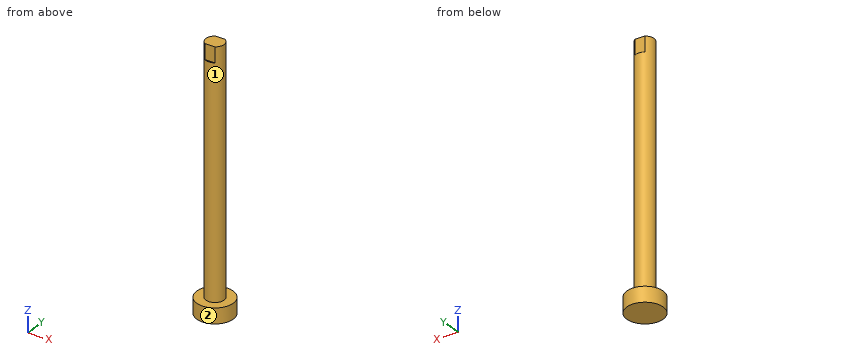
from build123d import *

# Parameters (mm, degrees)
F0_R     = 3
F1_DEPTH = 40
F2_R     = 6
F2_R_2   = 3
F3_DEPTH = 5
F5_DEPTH = 5


with BuildPart() as f1:
    # F0 (on Top) → F1 (new body, symmetric)
    with BuildSketch(Plane.XY):
        Circle(F0_R)
    extrude(amount=F1_DEPTH, both=True)

    # F2 (on face) → F3 (join)
    with BuildSketch(Plane(origin=(0, 0, -40), x_dir=(1, 0, 0), z_dir=(0, 0, -1))):
        Circle(F2_R)
        Circle(F2_R_2, mode=Mode.SUBTRACT)
        Circle(F2_R_2)
    extrude(amount=F3_DEPTH)

    # F4 (on face) → F5 (cut)
    with BuildSketch(Plane.XY.offset(40)):
        with BuildLine():
            Line((4.5341607578, -3.7982849256), (4.5341607578, -2.5))
            Line((4.5341607578, -2.5), (1.6583123952, -2.5))
            ThreePointArc((1.6583123952, -2.5), (0, -3), (-1.6583123952, -2.5))
            Line((-1.6583123952, -2.5), (-4.5341607578, -2.5))
            Line((-4.5341607578, -2.5), (-4.5341607578, -3.7982849256))
            Line((-4.5341607578, -3.7982849256), (4.5341607578, -3.7982849256))
        make_face()
        with BuildLine():
            ThreePointArc((-1.6583123952, -2.5), (0, -3), (1.6583123952, -2.5))
            Line((1.6583123952, -2.5), (-1.6583123952, -2.5))
        make_face()
        with BuildLine():
            Line((1.6583123952, 2.5), (4.5341607578, 2.5))
            Line((4.5341607578, 2.5), (4.5341607578, 3.7982849256))
            Line((4.5341607578, 3.7982849256), (-4.5341607578, 3.7982849256))
            Line((-4.5341607578, 3.7982849256), (-4.5341607578, 2.5))
            Line((-4.5341607578, 2.5), (-1.6583123952, 2.5))
            ThreePointArc((-1.6583123952, 2.5), (0, 3), (1.6583123952, 2.5))
        make_face()
        with BuildLine():
            Line((-1.6583123952, 2.5), (1.6583123952, 2.5))
            ThreePointArc((1.6583123952, 2.5), (0, 3), (-1.6583123952, 2.5))
        make_face()
    extrude(amount=-F5_DEPTH, mode=Mode.SUBTRACT)


solid = f1.part
The model under review builds one solid part; all positions refer to its coordinate system, in mm. Face numbers are marked on the shaded views. A direction names the side the tool comes from. Give positions to 0.01 mm unless a question says otherwise; leave off trailing zeros. Order: outer loops, then holes, each group sorted by start corner. A loop starts at its lowest first (then second) coordinate and runs counter-clockwise, first axis right, second up. Notation, with made-up numbers: M 68,37.5 L 109,37.5 A7 ccw 109,48.5 Z; hole C 85,49 d4. An arc over 180 degrees is marked long. Answer in a Markdown table with one row per item. Add a question column.
1. Add section C-C on z = -16. State the section outline as (x, y) points.
2. To check wall thickness, follow line 1 along Z through (x, y) = (-1.5, -4); line 2 along X through (y, z) = (2.5, 24); line 3 along X through (y, z) = (-0.25, -22). State the ranges of each line that lie inside material, in increasing order.
3. Add section B-B on x = 0. State the section outline as (y, z) points, plus the area to 3 significant figures.
4. For pin 1 Ø3.5 at (x, z) = (0.5, 38) entering from -Y; pin 2 Ø2.5 at (x, z) = (0, 38) entering from +Y; pin 3 Ø5 at (y, z) = (-0.5, 27.5) entering from +X, all flat-tipped, find the tip position at first contact; note any pin that passes through.
5. Machinability: for the marked faces 1 and 2, which of the approach directions +Z, -Z, +X, -X, +Y, -Y give a long, thin tool a straight path to every point of the face, cutting with its end or side? Answer none if there is none.
6. Add section A-A on y = 0. State the section outline as (x, z) points, plus the area to 3 significant figures.
7. Add section D-D on y = 4.75. State the section outline as (x, z) points, plus the area to 3 significant figures.
The answers:
| question | item | result |
|---|---|---|
| 1 | outline | C 0,0 d6 |
| 2 | line 1 | -45 to -40 |
| 2 | line 2 | -1.66 to 1.66 |
| 2 | line 3 | -2.99 to 2.99 |
| 3 | outline | M -6,-45 L 6,-45 L 6,-40 L 3,-40 L 3,35 L 2.5,35 L 2.5,40 L -2.5,40 L -2.5,35 L -3,35 L -3,-40 L -6,-40 Z |
| 3 | area | 535 mm2 |
| 4 | pin 1 | y = -2.5 |
| 4 | pin 2 | y = 2.5 |
| 4 | pin 3 | x = 3 |
| 5 | face 1 | +Z |
| 5 | face 2 | +Z, -Z |
| 6 | outline | M -6,-45 L 6,-45 L 6,-40 L 3,-40 L 3,40 L -3,40 L -3,-40 L -6,-40 Z |
| 6 | area | 540 mm2 |
| 7 | outline | M -3.67,-45 L 3.67,-45 L 3.67,-40 L -3.67,-40 Z |
| 7 | area | 36.7 mm2 |
